Design review of the part built by this model. Coordinates are the model's own, in mm. A direction names the side the tool comes from. Coordinates: 2 decimals unless noted, no trailing zeros. Write each loop counter-clockwise with the first axis right and the second up, starting at its lowest first coordinate (ties: lowest second). Pieces come first, ordered by that corner, then holes.
Q1. The part is to be moulded in two halves that separate along X. For faces 1 (the face through (43, 10, 20)), 2 (the face through (8, 6, 20)), 3 (the face through (1.3, 23.6, 32)), 4 (the face through (0, 40, 18)), say which applies: +X half, -X half, draft (parallel to the pull), parting line (faces both ways), or undercut.
Q2. Add section A-A, the plane x = 43.25. Give the boundary of the cut face in (y, z), plus the area to 3 significant figures.
Q3. Machinability: for faces 5 (the face through (39.5, 6, 20)), 6 (the face through (18.23, 1.27, 18.96)), 7 (the face through (48.23, 54.33, 31.97)), which of the approach directions +Z, -Z, +X, -X, +Y, -Y give a long, thin tool a straight path to every point of the face, cutting with its end or side? Answer none if there is none.
Q4. Add section D-D, the plane z = 33. Give the boundary of the cut face in (x, y).
Q5. Clearance check with flat-ended pins moving along their axes: pin 1 Ø2 at (x, z) = (23.419, 21.639) entering from +Y; pin 2 Ø2 at (y, z) = (22.95, 32.88) entering from -X; pin 3 Ø3 at (x, y) = (43.25, 6.25) entering from +Z; pin 4 Ø2.5 at (y, z) = (53, 32.667) entering from +X. State where each tip first meets the part, or that it passes through.
Q6. To check wall thickness, follow probe 1 along X at (y, z) = (6.25, 13); probe 2 along X at (y, z) = (72.75, 14); probe 3 along X at (y, z) = (38.5, 26.5). State the ranges of each line that lie inside material, in increasing order.
Q7. Add section B-B, the plane y = 6.25. Give the boundary of the cut face in (x, z), plus the area to 3 significant figures.
Q8. Add section C-C, the plane x = 13.25. Give the boundary of the cut face in (y, z).
Autodesk Inventor part; units mm, degrees
ref_plane "YZ Plane" through (0, 0, 0) normal (1, 0, 0) x (0, 1, 0)
ref_plane "XZ Plane" through (0, 0, 0) normal (0, 1, 0) x (-1, 0, 0)
ref_plane "XY Plane" through (0, 0, 0) normal (0, 0, 1) x (1, 0, 0)
sketch "Sketch1" plane through (0, 0, 0) normal (0, 0, 1) x (1, 0, 0)
  line L0 (0, 0) -> (49.5, 0)
  line L1 (49.5, 0) -> (49.5, 79)
  line L2 (49.5, 79) -> (0, 79)
  line L3 (0, 79) -> (0, 0)
  dimension "d0" = 49.5
  dimension "d1" = 79
extrude "Extrusion1" add sketch "Sketch1" along normal blind 35.867
sketch "Sketch2" plane through (0, 0, 35.867) normal (0, 0, 1) x (1, 0, 0)
  line L0 (0, 79) -> (0, 0) construction
  line L1 (49.5, 79) -> (0, 79) construction
  line L2 (49.5, 0) -> (49.5, 79) construction
  line L3 (0, 0) -> (49.5, 0) construction
  line L4 (2.5, 2.5) -> (47, 2.5)
  line L5 (47, 2.5) -> (47, 76.5)
  line L6 (47, 76.5) -> (2.5, 76.5)
  line L7 (2.5, 76.5) -> (2.5, 2.5)
  dimension "d4" = 2.5
  dimension "d5" = 2.5
  dimension "d6" = 2.5
  dimension "d7" = 2.5
extrude "Extrusion2" cut sketch "Sketch2" against normal blind 32.367
sketch "Sketch3" plane through (0, 0, 0) normal (0, -1, 0) x (1, 0, 0)
  line L0 (0, 0) -> (49.5, 0) construction
  line L1 (49.5, 0) -> (49.5, 35.867) construction
  line L2 (0, 35.867) -> (49.5, 35.867) construction
  line L3 (0, 0) -> (0, 35.867) construction
  point P0 (21.75, 18.5)
  point P1 (24.75, 35.867)
  dimension "d12" = 17.367
  dimension "d31" = 21.75
hole "Hole1" at (21.75, 0, 18.5) direction (0, 1, 0) diameter 7.1 depth 2.5
sketch "Sketch4" plane through (0, 0, 0) normal (0, -1, 0) x (1, 0, 0)
  circle A0 centre (21.75, 18.5) radius 3.55 construction
  line L0 (0, 0) -> (49.5, 0) construction
  line L1 (49.5, 0) -> (49.5, 35.867) construction
  line L2 (0, 35.867) -> (49.5, 35.867) construction
  line L3 (0, 0) -> (0, 35.867) construction
  point P0 (21.75, 27)
  dimension "d20" = 8.5
hole "Hole2" at (21.75, 0, 27) direction (0, 1, 0) diameter 3.3 depth 2.5
pattern_circular "Circular Pattern1" count 4 over 360 about axis through (21.75, 99.8884, 18.5) along (0, -1, 0) of "Hole2"
sketch "Sketch5" plane through (0, 0, 0) normal (-1, 0, 0) x (0, 0, 1)
  line L0 (35.867, 79) -> (35.867, 0)
  line L1 (0, 0) -> (35.867, 0)
  point P0 (32.881, 22.9529)
  point P1 (10.021, 53.4329)
  dimension "d32" = 2.986
  dimension "d33" = 30.48
  dimension "d34" = 22.86
  dimension "d35" = 22.9529
hole "Hole3" at (0, 22.9529, 32.881) at (0, 53.4329, 10.021) direction (1, 0, 0) diameter 2.184 depth 2.5
fillet "Fillet3" radius 2 3 edges at (24.75, 2.5, 3.5) (47, 2.5, 19.6835) (2.5, 2.5, 19.6835)
sketch "Sketch6" plane through (49.5, 0, 0) normal (1, 0, 0) x (0, 0, -1)
  line L0 (-35.867, 0) -> (-35.867, 79)
  line L1 (0, 79) -> (-35.867, 79)
  point P0 (0, 0)
  point P1 (-16.667, 23)
  point P2 (-32.667, 53)
  dimension "d44" = 30
  dimension "d47" = 26
  dimension "d55" = 3.2
  dimension "d56" = 16
hole "Hole4" at (49.5, 23, 16.667) at (49.5, 53, 32.667) direction (-1, 0, 0) diameter 3 depth 2.5
sketch "Sketch7" plane through (0, 0, 35.867) normal (0, 0, 1) x (1, 0, 0)
  line L0 (49.5, 0) -> (39.5, 0)
  line L1 (39.5, 0) -> (39.5, 10)
  line L2 (39.5, 10) -> (49.5, 10)
  line L3 (49.5, 10) -> (49.5, 0)
  line L4 (0, 0) -> (8, 0)
  line L5 (8, 0) -> (8, 10)
  line L6 (8, 10) -> (0, 10)
  line L7 (0, 10) -> (0, 0)
  line L8 (0, 79) -> (10, 79)
  line L9 (10, 79) -> (10, 69)
  line L10 (10, 69) -> (0, 69)
  line L11 (0, 69) -> (0, 79)
  line L12 (49.5, 79) -> (39.5, 79)
  line L13 (39.5, 79) -> (39.5, 69)
  line L14 (39.5, 69) -> (49.5, 69)
  line L15 (49.5, 69) -> (49.5, 79)
  line L16 (49.5, 79) -> (0, 79)
  line L17 (49.5, 0) -> (49.5, 79)
  point P0 (4, 0)
  point P1 (44.5, 0)
  point P2 (5, 79)
  point P3 (44.5, 79)
  point P4 (49.5, 74)
  point P5 (49.5, 5)
  point P6 (0, 74)
  point P7 (0, 5)
  point P8 (24.75, 79)
  point P9 (49.5, 39.5)
  dimension "d57" = 10
  dimension "d58" = 8
  dimension "d59" = 10
  dimension "d60" = 10
  dimension "d61" = 10
  dimension "d62" = 10
  dimension "d63" = 10
  dimension "d64" = 10
extrude "Extrusion3" add sketch "Sketch7" against normal up to surface (32.367 mm away)
sketch "Sketch8" plane through (0, 0, 35.867) normal (0, 0, 1) x (1, 0, 0)
  line L0 (39.5, 2.5) -> (8, 2.5) construction
  line L1 (8, 2.5) -> (8, 10) construction
  line L2 (8, 10) -> (2.5, 10) construction
  line L3 (2.5, 10) -> (2.5, 69) construction
  line L4 (2.5, 69) -> (10, 69) construction
  line L5 (10, 69) -> (10, 76.5) construction
  line L6 (10, 76.5) -> (39.5, 76.5) construction
  line L7 (39.5, 76.5) -> (39.5, 69) construction
  line L8 (39.5, 69) -> (47, 69) construction
  line L9 (47, 69) -> (47, 10) construction
  line L10 (47, 10) -> (39.5, 10) construction
  line L11 (39.5, 10) -> (39.5, 2.5) construction
  line L12 (49.5, 79) -> (0, 79) construction
  line L13 (0, 79) -> (0, 0) construction
  line L14 (0, 0) -> (49.5, 0) construction
  line L15 (49.5, 0) -> (49.5, 79) construction
  point P0 (5.25, 6.25)
  point P1 (43.25, 6.25)
  point P2 (43.25, 72.75)
  point P3 (6.25, 72.75)
  point P4 (5.25, 10)
  point P5 (8, 6.25)
  point P6 (39.5, 6.25)
  point P7 (39.5, 72.75)
  point P8 (10, 72.75)
  point P9 (6.25, 69)
  point P10 (43.25, 69)
  point P11 (43.25, 10)
hole "Hole5" at (5.25, 6.25, 35.867) at (43.25, 6.25, 35.867) at (43.25, 72.75, 35.867) at (6.25, 72.75, 35.867) direction (0, 0, -1) diameter 3.3 end through all
sketch "Sketch9" plane through (0, 79, 0) normal (0, 1, 0) x (1, 0, 0)
  line L0 (49.5, -35.867) -> (0, -35.867)
  point P0 (0, 0)
  point P1 (23.419, -21.639)
  point P2 (24.75, -35.867)
  point P3 (10, -35.867)
  dimension "d75" = 14.228
  dimension "d87" = 13.419
hole "Hole6" at (23.419, 79, 21.639) direction (0, -1, 0) diameter 3.3 depth 2.5
sketch "Sketch10" plane through (10, 76.5, 35.867) normal (0, -1, 0) x (1, 0, 0)
  line L0 (0, -32.367) -> (29.5, -32.367) construction
  circle A0 centre (13.419, -14.228) radius 1.65 construction
  line L1 (0, 0) -> (0, -32.367) construction
  line L2 (0, -32.367) -> (29.5, -32.367) construction
  line L3 (29.5, -32.367) -> (29.5, 0) construction
  line L4 (0, 0) -> (29.5, 0) construction
  line L5 (24.75, -32.367) -> (4.75, -32.367)
  line L6 (4.75, -32.367) -> (4.75, -29.367)
  line L7 (4.75, -29.367) -> (24.75, -29.367)
  line L8 (24.75, -29.367) -> (24.75, -32.367)
  point P0 (-10, -35.867)
  point P1 (14.75, -29.367)
  point P2 (14.75, 0)
  dimension "d83" = 20
  dimension "d84" = 3
extrude "Extrusion4" cut sketch "Sketch10" against normal through all
properties part number "Parte de abajo contenedor"
Here are the results:
1. face 1: undercut
1. face 2: undercut
1. face 3: draft
1. face 4: -X half
2. outline: (0, 0) - (4.6, 0) - (4.6, 35.87) - (0, 35.87) - close; (7.9, 0) - (71.1, 0) - (71.1, 35.87) - (69, 35.87) - (69, 3.5) - (10, 3.5) - (10, 35.87) - (7.9, 35.87) - close; (74.4, 0) - (79, 0) - (79, 35.87) - (74.4, 35.87) - close
2. area: 687 mm2
3. face 5: +Z
3. face 6: -Y
3. face 7: +X
4. outline: (0, 0) - (49.5, 0) - (49.5, 51.54) - (47, 51.54) - (47, 10) - (39.5, 10) - (39.5, 2.5) - (8, 2.5) - (8, 10) - (2.5, 10) - (2.5, 21.87) - (0, 21.87) - close; (0, 24.04) - (2.5, 24.04) - (2.5, 69) - (10, 69) - (10, 76.5) - (39.5, 76.5) - (39.5, 69) - (47, 69) - (47, 54.46) - (49.5, 54.46) - (49.5, 79) - (0, 79) - close; hole circle Ø3.3 at (5.25, 6.25); hole circle Ø3.3 at (6.25, 72.75); hole circle Ø3.3 at (43.25, 6.25); hole circle Ø3.3 at (43.25, 72.75)
5. pin 1: stops at y = 2.5
5. pin 2: stops at x = 47
5. pin 3: passes through
5. pin 4: stops at x = 2.5
6. probe 1: x = 0 to 3.6, 6.9 to 8, 39.5 to 41.6, 44.9 to 49.5
6. probe 2: x = 0 to 4.6, 7.9 to 10, 39.5 to 41.6, 44.9 to 49.5
6. probe 3: x = 0 to 2.5, 47 to 49.5
7. outline: (0, 0) - (3.6, 0) - (3.6, 35.87) - (0, 35.87) - close; (6.9, 0) - (41.6, 0) - (41.6, 35.87) - (39.5, 35.87) - (39.5, 3.5) - (8, 3.5) - (8, 35.87) - (6.9, 35.87) - close; (44.9, 0) - (49.5, 0) - (49.5, 35.87) - (44.9, 35.87) - close
7. area: 519 mm2
8. outline: (0, 0) - (79, 0) - (79, 35.87) - (76.5, 35.87) - (76.5, 3.5) - (4.5, 3.5) arc R2 cw to (2.5, 5.5) - (2.5, 16.85) - (0, 16.85) - close; (0, 20.15) - (2.5, 20.15) - (2.5, 35.87) - (0, 35.87) - close
